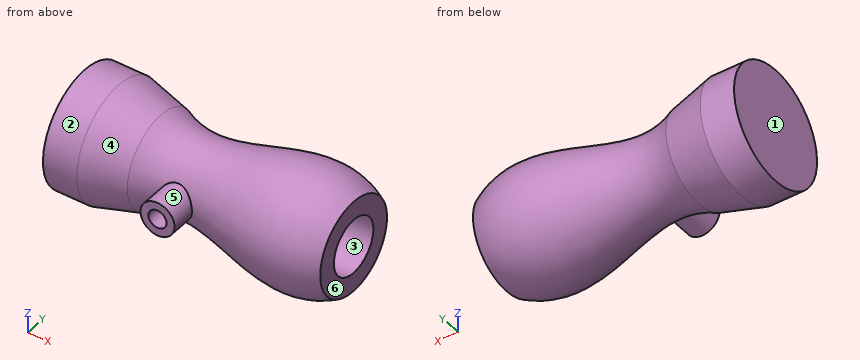
```python
from build123d import *

# Parameters (mm, degrees)
SKETCH_2_R           = 34.370841625
CUT_EXTRUDE_1_DEPTH  = 230
EXTRUDE_1_DEPTH      = 33
EXTRUDE_1_DEPTH_BACK = 10
SKETCH_3_R           = 21.25
SKETCH_3_R_2         = 11.25
SKETCH_4_R           = 72.26496
EXTRUDE_1_2_DEPTH    = 27


with BuildPart() as part:
    # 草圖1 → 旋轉1 (revolve)
    with BuildSketch(Plane.XY, mode=Mode.PRIVATE) as revolve_1_sk:
        with BuildLine():
            Line((0, 0), (0, 72.26496))
            Line((0, 72.26496), (15.231045419, 72.26496))
            Line((15.231045419, 72.26496), (68.107845419, 58.16448))
            add(Edge.make_bspline(
                [(68.107845419, 58.16448), (147.660376362, 17.815554571), (226.419832208, 105.291746385), (308.823182562, 58.16448)],
                knots=[0, 0, 0, 0, 1, 1, 1, 1], degree=3))
            Line((308.823182562, 58.16448), (308.823182562, 0))
            Line((308.823182562, 0), (0, 0))
        make_face()
    revolve(revolve_1_sk.sketch.rotate(Axis((0, 0, 0), (1, 0, 0)), 90), axis=Axis((0, 0, 0), (1, 0, 0)))

    # 草圖2 → 除料-伸長1 (cut)
    with BuildSketch(Plane(origin=(308.823182562, 0, 0), x_dir=(0, 0, -1), z_dir=(1, 0, 0))):
        Circle(SKETCH_2_R)
    extrude(amount=-CUT_EXTRUDE_1_DEPTH, mode=Mode.SUBTRACT)

    # 草圖3 → Extrude 1 (add, two sides: drawn at the far end of the back side and taken through both)
    with BuildSketch(Plane(origin=(0, -70, 0), x_dir=(1, 0, 0), z_dir=(0, 1, 0)).offset(-EXTRUDE_1_DEPTH_BACK)):
        with Locations((121.401340983, 0)):
            Circle(SKETCH_3_R)
        with Locations((121.401340983, 0)):
            Circle(SKETCH_3_R_2, mode=Mode.SUBTRACT)
    extrude(amount=EXTRUDE_1_DEPTH + EXTRUDE_1_DEPTH_BACK)

    # 草圖4 → Extrude 1 2 (add)
    with BuildSketch(Plane.ZY):
        Circle(SKETCH_4_R)
    extrude(amount=EXTRUDE_1_2_DEPTH)


solid = part.part
```
Design review of the part built by this model. Coordinates are the model's own, in mm. Face numbers are marked on the shaded views. A direction names the side the tool comes from. Round coordinates to 2 decimals unless told otherwise and drop trailing zeros. Write each loop counter-clockwise with the first axis right and the second up, starting at its lowest first coordinate (ties: lowest second). Pieces come first, ordered by that corner, then holes. Notation, with made-up numbers: (18, 44.25) -> (77, 44.25) arc R22 ccw to (77, 75.25) -> close; hole circle Ø3 at (63, 6.25). An arc over 180 degrees is marked (long way). Write item = value, one per line. Start each with the question number.
1) Clearance check with flat-ended pins moving along their axes: pin 1 (8 mm diameter, centred on x = 47, z = -20.5, fed in from -Y); pin 2 (10 mm diameter, centred on x = 216.5, z = -22, fed in from -Y); pin 3 (10 mm diameter, centred on x = 47.5, z = -28.5, fed in from -Y). State where each tip first meets the part, or that it passes through.
2) Tool access review of the marked faces 1 and 2: name each direction out of +Z, -Z, +X, -X, +Y, -Y from which nothing blocks a thin tool from reaching the whole face with its end or side.
3) Wall thickness on probe 1 along X at (y, z) = (23.5, 1); probe 2 along Y at (x, z) = (268, -9); probe 3 along Z at (x, y) = (111, -48): over which ranges is each line inside the solid? List them lowest first. Write a range as from..to.
4) Take a section at A-A, the plane x = 36. State the section outline as (y, z) points.
5) Mouldability with a two-part tool opening along X and no side actions: class the marked faces 3, 4, 5 and 6 as +X half, -X half, draft (parallel to the pull), parting line (faces both ways), or undercut.
Results list:
q1.pin_1 = -62.08
q1.pin_2 = -66.26
q1.pin_3 = -59.62
q2.face_1 = +Z, -Z, -X, +Y, -Y
q2.face_2 = -X
q3.probe_1 = -27..78.82
q3.probe_2 = -71.15..-33.17, 33.17..71.15
q3.probe_3 = -18.53..-4.29, 4.29..18.53
q4.outline = circle Ø133.45 at (0, 0)
q5.face_3 = draft
q5.face_4 = undercut
q5.face_5 = undercut
q5.face_6 = +X half
